from build123d import *

# Parameters (mm, degrees)
BOSS_EXTRUDE1_DEPTH = 7.62
CUT_EXTRUDE1_DEPTH  = 24.708556472


with BuildPart() as part:
    # Sketch1 → Boss-Extrude1 (new, symmetric)
    with BuildSketch(Plane.XY):
        with BuildLine():
            Line((-15.875, 0), (15.875, 0))
            ThreePointArc((15.875, 0), (0, 15.875), (-15.875, 0))
        make_face()
    extrude(amount=BOSS_EXTRUDE1_DEPTH, both=True)

    # Sketch2 → Cut-Extrude1 (cut, through all)
    with BuildSketch(Plane.XY):
        with BuildLine():
            Line((-13.426650235, 8.469987513), (-13.426650235, 3.198682523))
            Line((-13.426650235, 3.198682523), (11.508557344, 3.198682523))
            Line((11.508557344, 3.198682523), (11.508557344, 10.93474887))
            ThreePointArc((11.508557344, 10.93474887), (-1.56158004, 15.79800914), (-13.426650235, 8.469987513))
        make_face()
    extrude(amount=CUT_EXTRUDE1_DEPTH, mode=Mode.SUBTRACT)


solid = part.part
Geometry: final body of the model. Coordinates: model frame, mm. A direction names the side the tool comes from. Round coordinates to 2 decimals unless told otherwise and drop trailing zeros. Loops run counter-clockwise (first coordinate to the right, second up) from the corner with the lowest first, then second, coordinate; pieces in that order, holes last. Notation, with made-up numbers: M 82,-11 L 95,-11 A15 ccw 95,8 Z; hole C 48,16.5 d5. An arc over 180 degrees is marked long. Put each result on its own line as item: value. Start each with the question number.
(1) Section query C-C (y = 4.75). Return loops of the section in (x, z).
(2) Section query A-A (z = 1). Return loops of the section in (x, y) (3 decimals), then the cut area to 3 significant figures.
(3) Section query D-D (z = -3.5). Return loops of the section in (x, y) (3 decimals).
(4) Draft query along X for faces 1 (the face through (0, 0, 0)), 2 (the face through (0.35, 15.87, -1.59)), 3 (the face through (-1, 8, 0)). Return one class per face: +X half, -X half, draft (parallel to the pull), parting line (faces both ways), or undercut.
(5) Section query B-B (x = 0). Return loops of the section in (y, z) (3 decimals).
(6) Material intervals for line 1 along Y through (x, z) = (3.5, 7.25); line 2 along Z through (x, y) = (1.5, 7.25); line 3 along Y through (x, z) = (-11.5, -6.5), sorted ascending. Write a range as [from, to].
(7) Contact query for flat-ended pins moving along their axis: pin 1 Ø2 at (y, z) = (3, 2.5) entering from +X; pin 2 Ø1.5 at (x, z) = (8, 3) entering from +Y; pin 3 Ø6 at (x, y) = (-0.5, 10.5) entering from +Z; pin 4 Ø8 at (x, z) = (1.5, 3) entering from -Y. Output: stop coordinate, or through.
(8) Set-up query: faces 4 (the face through (11.509, 7, 4)), 5 (the face through (0, 6, -7.62)). Return all of +Z, -Z, +X, -X, +Y, -Y with unobstructed straight access to the full face (end or side cutting, diameter ignored); none if empty.
Findings below:
1. outline: M -15.15,-7.62 L 15.15,-7.62 L 15.15,7.62 L 11.51,7.62 L 11.51,0 L -13.43,0 L -13.43,7.62 L -15.15,7.62 Z
2. outline: M -15.875,0 L 15.875,0 A15.875 ccw 11.509,10.935 L 11.509,3.199 L -13.427,3.199 L -13.427,8.47 A15.875 ccw Z
2. area: 127 mm2
3. outline: M -15.875,0 L 15.875,0 A15.875 ccw Z
4. face 1: draft
4. face 2: parting line
4. face 3: undercut
5. outline: M 0,-7.62 L 15.875,-7.62 L 15.875,0 L 3.199,0 L 3.199,7.62 L 0,7.62 Z
6. line 1: y = [0, 3.2]
6. line 2: z = [-7.62, 0]
6. line 3: y = [0, 10.94]
7. pin 1: stops at x = 15.75
7. pin 2: stops at y = 3.2
7. pin 3: stops at z = 0
7. pin 4: stops at y = 0
8. face 4: +Z, +Y
8. face 5: -Z, +X, -X, +Y, -Y
